Read the model definition and answer for the solid it produces. Units are mm, in the model's axes. A direction names the side the tool comes from. Coordinates: 2 decimals unless noted, no trailing zeros. Write each loop counter-clockwise with the first axis right and the second up, starting at its lowest first coordinate (ties: lowest second). Pieces come first, ordered by that corner, then holes. Notation, with made-up numbers: M 36,-37 L 56,-37 A33 cw 56,-4 Z; hole C -33.75,86.25 d8. An arc over 180 degrees is marked long. Write item = value, one per line.
Solid Edge part; units mm, degrees
sketch "Sketch1" plane through (0, 0, 0) normal (0, -1, 0) x (1, 0, 0)
  line L0 (-125.8929, -60.4726) -> (-5.8929, -60.4726)
  line L1 (-5.8929, -60.4726) -> (-5.8929, 89.5274)
  line L2 (-5.8929, 89.5274) -> (-125.8929, 89.5274)
  line L3 (-125.8929, 89.5274) -> (-125.8929, -60.4726)
  dimension "D1" = 125.8929
  dimension "D2" = 5.8929
extrude "Protrusion1" add sketch "Sketch1" against normal blind 10
sketch "Sketch2" plane through (-70.8929, 0, 14.5274) normal (0, -1, 0) x (1, 0, 0)
  circle A0 centre (5, -10) radius 8
  circle A1 centre (5, -10) radius 12.5
extrude "ExtrudedCutout_1" cut sketch "Sketch2" against normal blind 1
sketch "Sketch3" plane through (-70.8929, 0, 4.5274) normal (0, -1, 0) x (1, 0, 0)
  circle A0 centre (5, 0) radius 7.5
extrude "Cutout1" cut sketch "Sketch3" against normal through all
sketch "Sketch4" plane through (-70.8929, 10, 14.5274) normal (0, 1, 0) x (-1, 0, 0)
  circle A0 centre (-5, 60) radius 5
  circle A1 centre (35, 60) radius 5
  circle A2 centre (-45, 60) radius 5
  dimension "D1" = 45
extrude "Cutout2" cut sketch "Sketch4" against normal through all
Item 1: Find section B-B (x = -104.5). Determine the outline of the cut face in (y, z).
Worked answers:
outline = M 0,-60.47 L 10,-60.47 L 10,69.73 L 0,69.73 Z; M 0,79.33 L 10,79.33 L 10,89.53 L 0,89.53 Z
Item 2: Find section A-A (z = 1.5). Determine the outline of the cut face in (x, y).
Worked answers:
outline = M -125.89,0 L -78.02,0 L -78.02,1 L -73.3,1 L -73.3,0 L -72.75,0 L -72.75,10 L -125.89,10 Z; M -59.03,0 L -58.49,0 L -58.49,1 L -53.77,1 L -53.77,0 L -5.89,0 L -5.89,10 L -59.03,10 Z
Item 3: Find section C-C (y = 4.5). Determine the outline of the cut face in (x, z).
Worked answers:
outline = M -125.89,-60.47 L -5.89,-60.47 L -5.89,89.53 L -125.89,89.53 Z; hole C -105.89,74.53 d10; hole C -65.89,4.53 d15; hole C -65.89,74.53 d10; hole C -25.89,74.53 d10
Item 4: Which of the six approach directions +Z, -Z, +X, -X, +Y, -Y give full straight-line access (tool end or side, diameter ignored) to faces 1 (the face through (-58.74, 4.93, 6.78)), 2 (the face through (-74.1, 1, 4.7))?
Worked answers:
face_1 = +Y, -Y
face_2 = -Y
Item 5: Consider line 1 along Z through (x, y) = (-26, 3.75); line 2 along X through (y, z) = (2, 4.5); line 3 along X through (y, z) = (3.25, 70.5). Determine where each line is inside the solid, lowest interval first. Write a range as from..to.
Worked answers:
line_1 = -60.47..69.53, 79.53..89.53
line_2 = -125.89..-73.39, -58.39..-5.89
line_3 = -125.89..-108.86, -102.93..-68.86, -62.93..-28.86, -22.93..-5.89
Item 6: For a pull along X with two mould halves and no side action, classify faces 3 (the face through (-104.809, 5.07, 69.646)), 4 (the face through (-5.893, 5, 13)), 5 (the face through (-72.24, 0.49, -0.34)), 6 (the face through (-65, 5, 89.527)) as released by +X, released by -X, zero draft, split by the parting line, or undercut.
Worked answers:
face_3 = undercut
face_4 = released by +X
face_5 = undercut
face_6 = zero draft
